```python
from build123d import *

# Parameters (mm, degrees)
SKETCH1_W             = 6
SKETCH1_H             = 6
SKETCH1_R             = 1
BOSS_EXTRUDE1_DEPTH   = 15
BOSS_EXTRUDE1_2_DEPTH = 15
BOSS_EXTRUDE1_3_DEPTH = 15
BOSS_EXTRUDE1_4_DEPTH = 15
SKETCH2_W             = 39.5
SKETCH2_H             = 33.999999999
BOSS_EXTRUDE2_DEPTH   = 1
SKETCH3_W             = 39.5
SKETCH3_H             = 33.999999999
BOSS_EXTRUDE3_DEPTH   = 22
SKETCH4_W             = 37.5
SKETCH4_H             = 17.999999999
CUT_EXTRUDE1_DEPTH    = 22
FILLET1_R             = 7
SKETCH7_W             = 6
SKETCH7_H             = 0.6
CUT_EXTRUDE2_DEPTH    = 4
SKETCH8_W             = 9.999999999
SKETCH8_H             = 6
CUT_EXTRUDE3_DEPTH    = 4
FILLET2_R             = 2
SKETCH9_W             = 10
SKETCH9_H             = 6
SKETCH9_W_2           = 9
CUT_EXTRUDE4_DEPTH    = 4
FILLET3_R             = 2
SKETCH10_W            = 10
SKETCH10_H            = 6
CUT_EXTRUDE5_DEPTH    = 4
FILLET4_R             = 2
SKETCH11_W            = 2
SKETCH11_H            = 2
CUT_EXTRUDE6_DEPTH    = 4


with BuildPart() as part:
    # Sketch1 → Boss-Extrude1 (new body)
    with BuildSketch(Plane(origin=(0, 0, 0), x_dir=(1, 0, 0), z_dir=(0, 1, 0))):
        with Locations((-7.839776389, 20.365683815)):
            Rectangle(SKETCH1_W, SKETCH1_H)
        with Locations(Location((-7.339776389, 19.865683815, 0), (0, 0, 270))):
            Circle(SKETCH1_R, mode=Mode.SUBTRACT)
    extrude(amount=BOSS_EXTRUDE1_DEPTH)



with BuildPart() as body_2:
    # Sketch1 → Boss-Extrude1 2 (new body)
    with BuildSketch(Plane(origin=(0, 0, 0), x_dir=(1, 0, 0), z_dir=(0, 1, 0))):
        with Locations((25.660223611, 20.365683814)):
            Rectangle(SKETCH1_W, SKETCH1_H)
        with Locations(Location((25.160223611, 19.865683814, 0), (0, 0, 270))):
            Circle(SKETCH1_R, mode=Mode.SUBTRACT)
    extrude(amount=BOSS_EXTRUDE1_2_DEPTH)


with BuildPart() as body_3:
    # Sketch1 → Boss-Extrude1 3 (new body)
    with BuildSketch(Plane(origin=(0, 0, 0), x_dir=(1, 0, 0), z_dir=(0, 1, 0))):
        with Locations((-7.839776389, -7.634316185)):
            Rectangle(SKETCH1_W, SKETCH1_H)
        with Locations(Location((-7.339776389, -7.134316185, 0), (0, 0, 270))):
            Circle(SKETCH1_R, mode=Mode.SUBTRACT)
    extrude(amount=BOSS_EXTRUDE1_3_DEPTH)


with BuildPart() as body_4:
    # Sketch1 → Boss-Extrude1 4 (new body)
    with BuildSketch(Plane(origin=(0, 0, 0), x_dir=(1, 0, 0), z_dir=(0, 1, 0))):
        with Locations((25.660371549, -7.634316185)):
            Rectangle(SKETCH1_W, SKETCH1_H)
        with Locations(Location((25.160371549, -7.134316185, 0), (0, 0, 270))):
            Circle(SKETCH1_R, mode=Mode.SUBTRACT)
    extrude(amount=BOSS_EXTRUDE1_4_DEPTH)


with BuildPart() as part_1:
    add(part.part)

    add(body_2.part)  # Boss-Extrude2 merges body 2

    add(body_3.part)  # Boss-Extrude2 merges body 3

    add(body_4.part)  # Boss-Extrude2 merges body 4
    # Sketch2 → Boss-Extrude2 (add)
    with BuildSketch(Plane.XZ):
        with Locations((8.910223611, -6.365683814)):
            Rectangle(SKETCH2_W, SKETCH2_H)
    extrude(amount=BOSS_EXTRUDE2_DEPTH)

    # Sketch3 → Boss-Extrude3 (add)
    with BuildSketch(Plane.XZ.offset(1)):
        Polygon((-11.839776389, 9.730248223), (-11.839776389, 11.634316185), (29.660223611, 11.634316185), (29.660223611, 9.730248223), (29.660223611, -24.365683814), (28.803720569, -24.365683814), (-10.696279431, -24.365683814), (-11.839776389, -24.365683814), align=None)
        with Locations((8.910223611, -6.365683814)):
            Rectangle(SKETCH3_W, SKETCH3_H, mode=Mode.SUBTRACT)
    extrude(amount=-BOSS_EXTRUDE3_DEPTH)

    # Sketch4 → Cut-Extrude1 (cut)
    with BuildSketch(Plane(origin=(0, 0, 0), x_dir=(1, 0, 0), z_dir=(0, 1, 0))):
        with Locations((9.910223611, 6.365683815)):
            Rectangle(SKETCH4_W, SKETCH4_H)
    extrude(amount=-CUT_EXTRUDE1_DEPTH, mode=Mode.SUBTRACT)

    # Fillet1
    fillet1_edges = [part_1.edges().sort_by_distance(p)[0] for p in [
        (-8.839776389, -0.5, 2.634316185),
        (-8.839776389, -0.5, -15.365683814),
        (28.660223611, -0.5, -15.365683814),
        (28.660223611, -0.5, 2.634316185),
    ]]
    fillet(fillet1_edges, radius=FILLET1_R)

    # Sketch7 → Cut-Extrude2 (cut)
    with BuildSketch(Plane(origin=(0, 15, 0), x_dir=(1, 0, 0), z_dir=(0, 1, 0))):
        with Locations((-7.839776389, 17.665683815)):
            Rectangle(SKETCH7_W, SKETCH7_H)
        with Locations((-7.839776389, -4.934316185)):
            Rectangle(SKETCH7_W, SKETCH7_H)
    extrude(amount=-CUT_EXTRUDE2_DEPTH, mode=Mode.SUBTRACT)

    # Sketch8 → Cut-Extrude3 (cut)
    with BuildSketch(Plane.ZY.offset(-28.660223611)):
        with Locations((-6.365683815, 18)):
            Rectangle(SKETCH8_W, SKETCH8_H)
    extrude(amount=-CUT_EXTRUDE3_DEPTH, mode=Mode.SUBTRACT)

    # Fillet2
    fillet2_edges = [part_1.edges().sort_by_distance(p)[0] for p in [
        (29.160223611, 15, -11.365683814),
        (29.160223611, 15, -1.365683815),
    ]]
    fillet(fillet2_edges, radius=FILLET2_R)

    # Sketch9 → Cut-Extrude4 (cut)
    with BuildSketch(Plane(origin=(0, 0, 10.634316185), x_dir=(-1, 0, 0), z_dir=(0, 0, -1))):
        with Locations((-14.660371549, 18)):
            Rectangle(SKETCH9_W, SKETCH9_H)
        with Locations((-0.660223611, 18)):
            Rectangle(SKETCH9_W_2, SKETCH9_H)
    extrude(amount=-CUT_EXTRUDE4_DEPTH, mode=Mode.SUBTRACT)

    # Fillet3
    fillet3_edges = [part_1.edges().sort_by_distance(p)[0] for p in [
        (19.660371549, 15, 11.134316185),
        (9.660371549, 15, 11.134316185),
        (5.160223611, 15, 11.134316185),
        (-3.839776389, 15, 11.134316185),
    ]]
    fillet(fillet3_edges, radius=FILLET3_R)

    # Sketch10 → Cut-Extrude5 (cut)
    with BuildSketch(Plane.XY.offset(-23.365683814)):
        with Locations((14.660223611, 18)):
            Rectangle(SKETCH10_W, SKETCH10_H)
    extrude(amount=-CUT_EXTRUDE5_DEPTH, mode=Mode.SUBTRACT)

    # Fillet4
    fillet4_edges = [part_1.edges().sort_by_distance(p)[0] for p in [
        (19.660223611, 15, -23.865683814),
        (9.660223611, 15, -23.865683814),
    ]]
    fillet(fillet4_edges, radius=FILLET4_R)

    # Sketch11 → Cut-Extrude6 (cut)
    with BuildSketch(Plane.XY.offset(-23.365683814)):
        with Locations((0.160223611, 17)):
            Rectangle(SKETCH11_W, SKETCH11_H)
    extrude(amount=-CUT_EXTRUDE6_DEPTH, mode=Mode.SUBTRACT)


solid = part_1.part
```
Design review of the part built by this model. Coordinates are the model's own, in mm. A direction names the side the tool comes from. Coordinates: 2 decimals unless noted, no trailing zeros. Loops run counter-clockwise (first coordinate to the right, second up) from the corner with the lowest first, then second, coordinate; pieces in that order, holes last.
Q1. We need section B-B on y = 13.5. State the section outline as (x, z) points.
Reported:
outline: (-11.84, -24.37) - (29.66, -24.37) - (29.66, 11.63) - (-11.84, 11.63) - close; hole (-10.84, -17.97) - (-4.84, -17.97) - (-4.84, -23.37) - (22.66, -23.37) - (22.66, -17.37) - (28.66, -17.37) - (28.66, 4.63) - (22.66, 4.63) - (22.66, 10.63) - (-4.84, 10.63) - (-4.84, 5.23) - (-10.84, 5.23) - close; hole circle Ø2 at (-7.34, -19.87); hole circle Ø2 at (-7.34, 7.13); hole circle Ø2 at (25.16, -19.87); hole circle Ø2 at (25.16, 7.13)
Q2. The part is to be moulded in two halves that separate along Z. For faces 6 (the face through (9, 10, -24.366)), 7 (the face through (28.66, 10, -6)), 8 (the face through (9.66, 19, -24)), say which applies: +Z half, -Z half, draft (parallel to the pull), parting line (faces both ways), or undercut.
Reported:
face 6: -Z half
face 7: undercut
face 8: draft
Q3. Tool access review of faces 1 (the face through (0, 16, -24)), 2 (the face through (26.555, -0.507, 0.638)), 3 (the face through (29.66, 10, -7)), 4 (the face through (15, 15, -24)), 5 (the face through (-8, 13, -17.966)): name each direction out of +Z, -Z, +X, -X, +Y, -Y from which nothing blocks a thin tool from reaching the whole face with its end or side.
Reported:
face 1: +Z, -Z
face 2: +Y, -Y
face 3: +Z, -Z, +X, +Y, -Y
face 4: +Z, -Z, +Y
face 5: +Y
Q4. We need section A-A on x = 6.5. State the section outline as (y, z) points.
Reported:
outline: (-1, -24.37) - (21, -24.37) - (21, -23.37) - (0, -23.37) - (0, -15.37) - (-1, -15.37) - close; (-1, 2.63) - (0, 2.63) - (0, 10.63) - (21, 10.63) - (21, 11.63) - (-1, 11.63) - close
Q5. We need section C-C on z = -16.5. State the section outline as (x, y) points.
Reported:
outline: (-11.84, -1) - (29.66, -1) - (29.66, 21) - (28.66, 21) - (28.66, 0) - (-10.84, 0) - (-10.84, 21) - (-11.84, 21) - close
Q6. We need section D-D on x = 2. State the section outline as (y, z) points.
Reported:
outline: (-1, -24.37) - (21, -24.37) - (21, -23.37) - (0, -23.37) - (0, -15.37) - (-1, -15.37) - close; (-1, 2.63) - (0, 2.63) - (0, 10.63) - (15, 10.63) - (15, 11.63) - (-1, 11.63) - close
Q7. For pin 1 (0.6 mm diameter, centred on x = 25, z = -19.5, fed in from +Y); pin 2 (0.8 mm diameter, centred on x = -0.5, z = 11, fed in from +Y), all flat-tipped, find the tip position at first contact; note any pin that passes through.
Reported:
pin 1: stops at y = 0
pin 2: stops at y = 15
Q8. To check wall thickness, follow line 1 (X direction, y = 14.5, z = 7); line 2 (Z direction, x = 9, y = 13.75); line 3 (X direction, y = 7.75, z = -15). State the ranges of each line that lie inside material, in increasing order.
Reported:
line 1: x = -11.84 to -8.33, -6.35 to -4.84, 22.66 to 24.17, 26.15 to 29.66
line 2: z = -24.37 to -23.37, 10.63 to 11.63
line 3: x = -11.84 to -10.84, 28.66 to 29.66
